Here's how the part is built. I have some questions about the finished solid (model axes, mm). A direction names the side the tool comes from. Round coordinates to 2 decimals unless told otherwise and drop trailing zeros. Loops run counter-clockwise (first coordinate to the right, second up) from the corner with the lowest first, then second, coordinate; pieces in that order, holes last. Notation, with made-up numbers: (89.25, -16) -> (110.25, -16) arc R30 cw to (110.25, 12) -> close; hole circle Ø1 at (83, 82). An arc over 180 degrees is marked (long way). Use one line per item in the form item = value. Start each with the question number.
Item 1: If we section it at B-B (x = -55): Write out the boundary of the cut face in (y, z).
Item 2: If I drill on L1, parallel to Z at x = -48, y = 49; L2, parallel to X at y = 26.5, z = 6; L3, parallel to Y at x = -9.5, z = 40, over which ranges is the centre line in solid material (lowest first)? Write a range as [from, to].
Item 3: If we section it at C-C (y = 29): Write out the boundary of the cut face in (x, z), then the cut area to 3 significant figures.
Item 4: Thinking about a two-plate mould opening in Z: for faces 1 (the face through (-40, 45, 5)), 2 (the face through (-41, 41, 80)), 3 (the face through (-70, 3, 41)), which applies, released by +Z, released by -Z, zero draft, split by the parting line, or undercut?
Item 5: For faces 4 (the face through (-5, 0, 39)), 5 (the face through (-40, 10, 78)), 6 (the face through (-40, 45, 75)), which set-ups out of +Z, -Z, +X, -X, +Y, -Y let a thin tool reach every point of the face, with its end or its side?
Item 6: If we section it at A-A (z = 28): Write out the boundary of the cut face in (x, y), then the cut area to 3 significant figures.
Item 7: I'm going to push flat-ended pins straight in: pin 1 Ø2 at (y, z) = (20.5, 57.5) entering from +X; pin 2 Ø1.5 at (x, z) = (-8.5, 34) entering from +Y; pin 3 Ø4 at (x, z) = (-24, 78) entering from -Y. Where does each tip first touch, or does it pass through?
```python
from build123d import *

# Parameters (mm, degrees)
SKETCH1_W           = 80
SKETCH1_H           = 80
BOSS_EXTRUDE1_DEPTH = 80
CUT_EXTRUDE1_DEPTH  = 114
SKETCH3_W           = 70
SKETCH3_H           = 70
CUT_EXTRUDE3_DEPTH  = 70


with BuildPart() as part:
    # Sketch1 → Boss-Extrude1 (new body)
    with BuildSketch(Plane.XY):
        with Locations((-40, 40)):
            Rectangle(SKETCH1_W, SKETCH1_H)
    extrude(amount=BOSS_EXTRUDE1_DEPTH)

    # Sketch2 → Cut-Extrude1 (cut)
    with BuildSketch(Plane.XY.offset(80)):
        Polygon((-70, 5), (-70, 0), (-10, 0), (-10, 5), (-5, 5), (-5, 10), (-75, 10), (-75, 5), align=None)
    extrude(amount=-CUT_EXTRUDE1_DEPTH, mode=Mode.SUBTRACT)

    # Sketch3 → Cut-Extrude3 (cut)
    with BuildSketch(Plane(origin=(0, 80, 0), x_dir=(1, 0, 0), z_dir=(0, 1, 0))):
        with Locations((-40, -40)):
            Rectangle(SKETCH3_W, SKETCH3_H)
    extrude(amount=-CUT_EXTRUDE3_DEPTH, mode=Mode.SUBTRACT)


solid = part.part
```
Values found:
q1.outline = (10, 0) -> (80, 0) -> (80, 5) -> (10, 5) -> close; (10, 75) -> (80, 75) -> (80, 80) -> (10, 80) -> close
q2.L1 = [0, 5], [75, 80]
q2.L2 = [-80, -75], [-5, 0]
q2.L3 = [0, 5]
q3.outline = (-80, 0) -> (0, 0) -> (0, 80) -> (-80, 80) -> close; hole (-75, 5) -> (-5, 5) -> (-5, 75) -> (-75, 75) -> close
q3.area = 1,500 mm2
q4.face_1 = undercut
q4.face_2 = released by +Z
q4.face_3 = zero draft
q5.face_4 = +Z, -Z, +X, -X, -Y
q5.face_5 = +Z, -Z
q5.face_6 = +Y
q6.outline = (-80, 0) -> (-70, 0) -> (-70, 5) -> (-75, 5) -> (-75, 80) -> (-80, 80) -> close; (-10, 0) -> (0, 0) -> (0, 80) -> (-5, 80) -> (-5, 5) -> (-10, 5) -> close
q6.area = 850 mm2
q7.pin_1 = 0
q7.pin_2 = 5
q7.pin_3 = 10
